Autodesk Inventor part; units mm, degrees
ref_plane "YZ Plane" through (0, 0, 0) normal (1, 0, 0) x (0, 1, 0)
ref_plane "XZ Plane" through (0, 0, 0) normal (0, 1, 0) x (-1, 0, 0)
ref_plane "XY Plane" through (0, 0, 0) normal (0, 0, 1) x (1, 0, 0)
sketch "Sketch1" plane through (0, 0, 0) normal (0, 1, 0) x (-1, 0, 0)
  line L0 (0, 0) -> (8, 0)
  line L1 (8, 0) -> (8, -10)
  line L2 (0, -10) -> (0, 0)
  line L3 (3.8, -10) -> (3.8, -6.2)
  line L4 (3.8, -6.2) -> (2, -6.2)
  line L5 (2, -6.2) -> (2, -10)
  line L6 (8, -10) -> (3.8, -10)
  line L7 (2, -10) -> (0, -10)
  dimension "d0" = 1.8
  dimension "d1" = 2
  dimension "d2" = 8
  dimension "d3" = 3.8
  dimension "d4" = 3.8
  dimension "d5" = 10
extrude "Extrusion1" add sketch "Sketch1" along normal blind 20
chamfer "Chamfer1" distance 0.25 angle 45 2 edges at (-2, 10, -10) (-3.8, 10, -10)
fillet "Fillet1" radius 1 4 edges at (-4, 20, 0) (-4, 0, 0) (-8, 10, -10) (0, 10, -10)
sketch "Sketch2" plane through (0, 20, 0) normal (0, 1, 0) x (1, 0, 0)
  arc A0 (0, 9) -> (-1, 10) centre (-1, 9) ccw
  line L0 (-1, 10) -> (-1.75, 10)
  line L1 (-2, 9.75) -> (-1.75, 10)
  line L2 (-2, 9.75) -> (-2, 6.2)
  line L3 (-2, 6.2) -> (-3.8, 6.2)
  line L4 (-3.8, 6.2) -> (-3.8, 9.75)
  line L5 (-4.05, 10) -> (-3.8, 9.75)
  line L6 (-4.05, 10) -> (-7, 10)
  arc A1 (-7, 10) -> (-8, 9) centre (-7, 9) ccw
  line L7 (-8, 9) -> (-8, 1)
  line L8 (0, 1) -> (-8, 1)
  line L9 (0, 1) -> (0, 9)
  circle A2 centre (-3.8, 6.2) radius 0.25
  circle A3 centre (-2, 6.2) radius 0.25
  point P0 (0, 0)
  dimension "d12" = 0.5
extrude "Extrusion2" cut sketch "Sketch2" against normal through all contours A3 L3 L2 | L2 L3 A3 | A2 L4 L3 | L3 L4 A2
fillet "Fillet2" radius 0.5 4 edges at (-3.55, 10, -6.2) (-3.8, 10, -6.45) (-2, 10, -6.45) (-2.25, 10, -6.2)
properties part number "capSenseHolder"
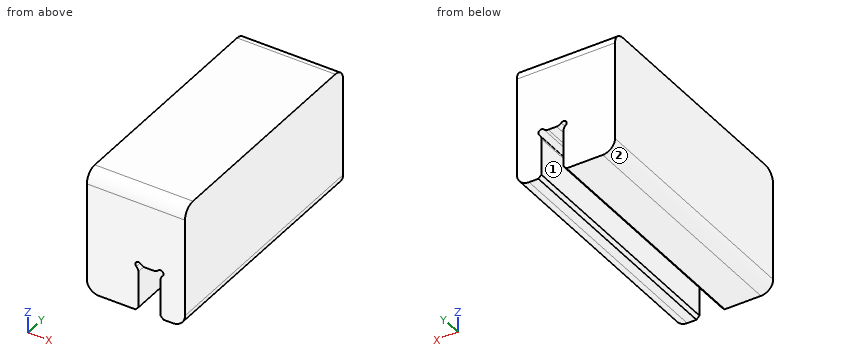
Here's how the part is built. I have some questions about the finished solid (model axes, mm). Face numbers are marked on the shaded views. A direction names the side the tool comes from. Round coordinates to 2 decimals unless told otherwise and drop trailing zeros. Write each loop counter-clockwise with the first axis right and the second up, starting at its lowest first coordinate (ties: lowest second). Pieces come first, ordered by that corner, then holes.
1. Suppose I cut it at C-C (y = 14.75). List the corners of the cut face in (x, z) for me, and give its area (3 significant figures).
2. Will this pin go through, and if not, where does the flat tip stop? pin 1 Ø1 at (x, y) = (-3.5, 13) entering from -Z.
3. Suppose I cut it at B-B (x = -3). List the corners of the cut face in (y, z) for me, and give its area (3 significant figures).
4. Suppose I cut it at A-A (z = -8.75). List the corners of the cut face in (x, y) for me.
5. For the marked faces 1 and 2, which set-ups out of +Z, -Z, +X, -X, +Y, -Y let a thin tool reach every point of the face, with its end or its side?
6. I need wall thicknesses on L1, parallel to X at y = 3.5, z = -9; L2, parallel to X at y = 16, z = -6; L3, parallel to Z at x = -2.5, y = 12. Which ranges of each line are inside material? Lowest first, please.
7. Suppose I cut it at D-D (x = -0.25). List the corners of the cut face in (y, z) for me, and give its area (3 significant figures).
Answer sheet:
1. outline: (-8, -9) arc R1 ccw to (-7, -10) - (-4.05, -10) - (-3.8, -9.75) - (-3.8, -6.76) arc R0.5 ccw to (-3.97, -6.39) arc R0.25 cw (long way) to (-3.61, -6.03) arc R0.5 ccw to (-3.24, -6.2) - (-2.56, -6.2) arc R0.5 ccw to (-2.19, -6.03) arc R0.25 cw (long way) to (-1.83, -6.39) arc R0.5 ccw to (-2, -6.76) - (-2, -9.75) - (-1.75, -10) - (-1, -10) arc R1 ccw to (0, -9) - (0, 0) - (-8, 0) - close
1. area: 72.3 mm2
2. pin 1: stops at z = -9.95
3. outline: (0, -6.2) - (20, -6.2) - (20, -1) arc R1 ccw to (19, 0) - (1, 0) arc R1 ccw to (0, -1) - close
3. area: 124 mm2
4. outline: (-8, 0) - (-3.8, 0) - (-3.8, 20) - (-8, 20) - close; (-2, 0) - (0, 0) - (0, 20) - (-2, 20) - close
5. face 1: -Z, +Y, -Y
5. face 2: -Z, -X, +Y, -Y
6. L1: x = -8 to -3.8, -2 to 0
6. L2: x = -8 to -3.95, -3.65 to -2.15, -1.85 to 0
6. L3: z = -6.2 to 0
7. outline: (0, -9.66) - (20, -9.66) - (20, -1) arc R1 ccw to (19, 0) - (1, 0) arc R1 ccw to (0, -1) - close
7. area: 193 mm2
